Solid Edge part; units mm, degrees
sketch "Sketch1" plane through (0, 0, 0) normal (0, -1, 0) x (1, 0, 0)
  line L0 (0, 30.3) -> (0, 0)
  line L1 (0, 0) -> (10, 0)
  line L2 (10, 0) -> (10, 20.3)
  line L3 (10, 20.3) -> (30.3, 20.3)
  line L4 (30.3, 20.3) -> (30.3, 0)
  line L5 (30.3, 0) -> (40.3, 0)
  line L6 (40.3, 0) -> (40.3, 20.3)
  line L7 (40.3, 20.3) -> (60.6, 20.3)
  line L8 (60.6, 20.3) -> (60.6, 0)
  line L9 (60.6, 0) -> (70.6, 0)
  line L10 (70.6, 0) -> (70.6, 30.3)
  line L11 (70.6, 30.3) -> (0, 30.3)
extrude "Protrusion1" add sketch "Sketch1" along normal blind 50
fillet "Round1" radius 10 2 edges at (0, -25, 30.3) (70.6, -25, 30.3)
fillet "Round2" radius 4.8 4 edges at (10, -25, 0) (30.3, -25, 0) (40.3, -25, 0) (60.6, -25, 0)
Source: CAD feature listing. Evaluate the final solid. Frame: model axes, mm. A direction names the side the tool comes from. Give positions to 0.01 mm unless a question says otherwise; leave off trailing zeros. Loops run counter-clockwise (first coordinate to the right, second up) from the corner with the lowest first, then second, coordinate; pieces in that order, holes last. Notation, with made-up numbers: (-32, -34) - (15, -34) arc R16 cw to (15, -21) - close; hole circle Ø7 at (67.25, 4.5). An arc over 180 degrees is marked (long way). Use CSV: the item, a comma, the result in double quotes.
1) Line query: line 1 (X direction, y = -13.5, z = 17); line 2 (X direction, y = -17, z = 2); line 3 (Z direction, x = 19, y = -4). Output: solid intervals per line, ascending.
Worked out:
line 1,"x = 0 to 10, 30.3 to 40.3, 60.6 to 70.6"
line 2,"x = 0 to 9.1, 31.2 to 39.4, 61.5 to 70.6"
line 3,"z = 20.3 to 30.3"
2) Cut plane C-C (x = 56). Output: boundary loops of the cut face in (y, z), and give its area (3 significant figures).
Worked out:
outline,"(-50, 20.3) - (0, 20.3) - (0, 30.3) - (-50, 30.3) - close"
area,"500 mm^2"
3) Set-up query: faces 1 (the flat face through (36, -25, 30.3)), 2 (the flat face through (40.3, -25, 12)). Return all of +Z, -Z, +X, -X, +Y, -Y with unobstructed straight access to the full face (end or side cutting, diameter ignored); none if empty.
Worked out:
face 1,"+Z, +X, -X, +Y, -Y"
face 2,"-Z, +Y, -Y"
4) Cut plane D-D (z = 3.5). Output: boundary loops of the cut face in (x, y).
Worked out:
outline,"(0, -50) - (9.82, -50) - (9.82, 0) - (0, 0) - close; (30.48, -50) - (40.12, -50) - (40.12, 0) - (30.48, 0) - close; (60.78, -50) - (70.6, -50) - (70.6, 0) - (60.78, 0) - close"
5) Cut plane B-B (y = -13.5). Output: boundary loops of the cut face in (x, z), and give its area (3 significant figures).
Worked out:
outline,"(0, 0) - (5.2, 0) arc R4.8 ccw to (10, 4.8) - (10, 20.3) - (30.3, 20.3) - (30.3, 4.8) arc R4.8 ccw to (35.1, 0) - (35.5, 0) arc R4.8 ccw to (40.3, 4.8) - (40.3, 20.3) - (60.6, 20.3) - (60.6, 4.8) arc R4.8 ccw to (65.4, 0) - (70.6, 0) - (70.6, 20.3) arc R10 ccw to (60.6, 30.3) - (10, 30.3) arc R10 ccw to (0, 20.3) - close"
area,"1,250 mm^2"
6) Pin query (flat end, axial travel): P1, Ø10, axis at x = 19.5, y = -37.5, coming from the -Z side. Return the tip coordinate at first contact, or that it passes through.
Worked out:
P1,"stops at z = 20.3"
7) Mould query, pull axis X, two halves, no side actions, for faces 3 (the cylindrical face through (3.01, -25.35, 27.45)), 4 (the flat face through (10, -25, 12)), 5 (the flat face through (30.3, -25, 13)), 6 (the flat face through (68, -25, 0)). Classes: +X half, -X half, draft (parallel to the pull), parting line (faces both ways), or undercut.
Worked out:
face 3,"-X half"
face 4,"undercut"
face 5,"undercut"
face 6,"draft"
8) Cut plane A-A (z = 11.5). Output: boundary loops of the cut face in (x, y).
Worked out:
outline,"(0, -50) - (10, -50) - (10, 0) - (0, 0) - close; (30.3, -50) - (40.3, -50) - (40.3, 0) - (30.3, 0) - close; (60.6, -50) - (70.6, -50) - (70.6, 0) - (60.6, 0) - close"
